```python
from build123d import *

# Parameters (mm, degrees)
CYLINDER017_R           = 1.4
CYLINDER017_DEPTH       = 210
CYLINDER017_PITCH_ANGLE = 90
CYLINDER016_R           = 1.4
CYLINDER016_DEPTH       = 16
CYLINDER016_PITCH_ANGLE = 90
CYLINDER022_R           = 1.4
CYLINDER022_DEPTH       = 210
CYLINDER022_PITCH_ANGLE = 90
CYLINDER011_R           = 1.4
CYLINDER011_DEPTH       = 140
CYLINDER018_R           = 1.4
CYLINDER018_DEPTH       = 16
CYLINDER013_R           = 1.4
CYLINDER013_DEPTH       = 140
CYLINDER020_R           = 1.4
CYLINDER020_DEPTH       = 16
CYLINDER014_R           = 1.4
CYLINDER014_DEPTH       = 140
CYLINDER019_R           = 1.4
CYLINDER019_DEPTH       = 16
CYLINDER021_R           = 1.4
CYLINDER021_DEPTH       = 16
CYLINDER012_R           = 1.4
CYLINDER012_DEPTH       = 140
CYLINDER015_R           = 1.4
CYLINDER015_DEPTH       = 210
CYLINDER015_PITCH_ANGLE = 90
CYLINDER002_R           = 12
CYLINDER002_DEPTH       = 40
BOX014_W                = 204
BOX014_H                = 20
BOX014_DEPTH            = 134
THICKNESS_T             = -6
FILLET007_R             = 3
BOX011_W                = 186
BOX011_H                = 34
BOX011_DEPTH            = 94
BOX010_W                = 192
BOX010_H                = 9
BOX010_DEPTH            = 122
BOX009_W                = 174
BOX009_H                = 10
BOX009_DEPTH            = 77
BOX012_W                = 192
BOX012_H                = 19
BOX012_DEPTH            = 21
BOX002_W                = 200
BOX002_H                = 40
BOX002_DEPTH            = 130
FILLET005_R             = 5
CYLINDER001_R           = 15
CYLINDER001_DEPTH       = 28
FILLET008_R             = 1
CHAMFER_SIZE            = 4
FILLET009_R             = 2


with BuildPart() as cylinder017:
    # Cylinder017 → Cylinder017 (new body)
    with BuildSketch(Plane.XY):
        Circle(CYLINDER017_R)
    extrude(amount=CYLINDER017_DEPTH)


with BuildPart() as cylinder017_1:
    # Cylinder017 pitch: moved
    add(cylinder017.part.rotate(Axis((0, 0, 0), (0, 1, 0)), CYLINDER017_PITCH_ANGLE))


with BuildPart() as cylinder017_2:
    # Cylinder017 placement: moved
    add(cylinder017_1.part.moved(Location((-5, 55, 65))))


with BuildPart() as cylinder016:
    # Cylinder016 → Cylinder016 (new body)
    with BuildSketch(Plane.XY):
        Circle(CYLINDER016_R)
    extrude(amount=CYLINDER016_DEPTH)


with BuildPart() as cylinder016_1:
    # Cylinder016 pitch: moved
    add(cylinder016.part.rotate(Axis((0, 0, 0), (0, 1, 0)), CYLINDER016_PITCH_ANGLE))


with BuildPart() as cylinder016_2:
    # Cylinder016 placement: moved
    add(cylinder016_1.part.moved(Location((-5, 55, 115))))


with BuildPart() as cylinder022:
    # Cylinder022 → Cylinder022 (new body)
    with BuildSketch(Plane.XY):
        Circle(CYLINDER022_R)
    extrude(amount=CYLINDER022_DEPTH)


with BuildPart() as cylinder022_1:
    # Cylinder022 pitch: moved
    add(cylinder022.part.rotate(Axis((0, 0, 0), (0, 1, 0)), CYLINDER022_PITCH_ANGLE))


with BuildPart() as cylinder022_2:
    # Cylinder022 placement: moved
    add(cylinder022_1.part.moved(Location((189, 55, 115))))


with BuildPart() as cylinder011:
    # Cylinder011 → Cylinder011 (new body)
    with BuildSketch(Plane(origin=(15, 55, 116), x_dir=(1, 0, 0), z_dir=(0, 0, 1))):
        Circle(CYLINDER011_R)
    extrude(amount=CYLINDER011_DEPTH)


with BuildPart() as cylinder018:
    # Cylinder018 → Cylinder018 (new body)
    with BuildSketch(Plane(origin=(15, 55, -5), x_dir=(1, 0, 0), z_dir=(0, 0, 1))):
        Circle(CYLINDER018_R)
    extrude(amount=CYLINDER018_DEPTH)


with BuildPart() as cylinder013:
    # Cylinder013 → Cylinder013 (new body)
    with BuildSketch(Plane(origin=(70, 55, 116), x_dir=(1, 0, 0), z_dir=(0, 0, 1))):
        Circle(CYLINDER013_R)
    extrude(amount=CYLINDER013_DEPTH)


with BuildPart() as cylinder020:
    # Cylinder020 → Cylinder020 (new body)
    with BuildSketch(Plane(origin=(125, 55, -5), x_dir=(1, 0, 0), z_dir=(0, 0, 1))):
        Circle(CYLINDER020_R)
    extrude(amount=CYLINDER020_DEPTH)


with BuildPart() as cylinder014:
    # Cylinder014 → Cylinder014 (new body)
    with BuildSketch(Plane(origin=(125, 55, 116), x_dir=(1, 0, 0), z_dir=(0, 0, 1))):
        Circle(CYLINDER014_R)
    extrude(amount=CYLINDER014_DEPTH)


with BuildPart() as cylinder019:
    # Cylinder019 → Cylinder019 (new body)
    with BuildSketch(Plane(origin=(70, 55, -5), x_dir=(1, 0, 0), z_dir=(0, 0, 1))):
        Circle(CYLINDER019_R)
    extrude(amount=CYLINDER019_DEPTH)


with BuildPart() as cylinder021:
    # Cylinder021 → Cylinder021 (new body)
    with BuildSketch(Plane(origin=(180, 55, -5), x_dir=(1, 0, 0), z_dir=(0, 0, 1))):
        Circle(CYLINDER021_R)
    extrude(amount=CYLINDER021_DEPTH)


with BuildPart() as cylinder012:
    # Cylinder012 → Cylinder012 (new body)
    with BuildSketch(Plane(origin=(180, 55, 116), x_dir=(1, 0, 0), z_dir=(0, 0, 1))):
        Circle(CYLINDER012_R)
    extrude(amount=CYLINDER012_DEPTH)


with BuildPart() as fusion009:
    # Cylinder015 → Cylinder015 (new body)
    with BuildSketch(Plane.XY):
        Circle(CYLINDER015_R)
    extrude(amount=CYLINDER015_DEPTH)


with BuildPart() as fusion009_1:
    # Cylinder015 pitch: moved
    add(fusion009.part.rotate(Axis((0, 0, 0), (0, 1, 0)), CYLINDER015_PITCH_ANGLE))


with BuildPart() as fusion009_2:
    # Cylinder015 placement: moved
    add(fusion009_1.part.moved(Location((-5, 55, 15))))

    # Fusion009: union Cylinder017, Cylinder016, Cylinder022, Cylinder011, Cylinder018, Cylinder013, Cylinder020, Cylinder014, Cylinder019, Cylinder021, Cylinder012
    add(cylinder017_2.part)
    add(cylinder016_2.part)
    add(cylinder022_2.part)
    add(cylinder011.part)
    add(cylinder018.part)
    add(cylinder013.part)
    add(cylinder020.part)
    add(cylinder014.part)
    add(cylinder019.part)
    add(cylinder021.part)
    add(cylinder012.part)


with BuildPart() as cylinder002:
    # Cylinder002 → Cylinder002 (new body)
    with BuildSketch(Plane(origin=(40, 70, 120), x_dir=(1, 0, 0), z_dir=(0, 0, 1))):
        Circle(CYLINDER002_R)
    extrude(amount=CYLINDER002_DEPTH)


with BuildPart() as fillet007:
    # Box014 → Box014 (new body)
    with BuildSketch(Plane(origin=(-2, 48, -2), x_dir=(1, 0, 0), z_dir=(0, 0, 1))):
        with Locations((102, 10)):
            Rectangle(BOX014_W, BOX014_H)
    extrude(amount=BOX014_DEPTH)

    # Thickness
    thickness_openings = [fillet007.faces().sort_by_distance(p)[0] for p in [
        (100, 48, 65),
        (100, 68, 65),
    ]]
    offset(amount=THICKNESS_T, openings=thickness_openings)

    # Fillet007
    fillet007_edges = [fillet007.edges().sort_by_distance(p)[0] for p in [
        (196, 58, 4),
        (4, 58, 4),
        (196, 58, 126),
        (4, 58, 126),
    ]]
    fillet(fillet007_edges, radius=FILLET007_R)


with BuildPart() as fillet007_1:
    # Fillet007 placement: moved
    add(fillet007.part.moved(Location((0, -8, 0))))


with BuildPart() as cube011:
    # Box011 → Box011 (new body)
    with BuildSketch(Plane(origin=(7, 45, 7), x_dir=(1, 0, 0), z_dir=(0, 0, 1))):
        with Locations((93, 17)):
            Rectangle(BOX011_W, BOX011_H)
    extrude(amount=BOX011_DEPTH)


with BuildPart() as cube010:
    # Box010 → Box010 (new body)
    with BuildSketch(Plane(origin=(4, 82, 4), x_dir=(1, 0, 0), z_dir=(0, 0, 1))):
        with Locations((96, 4.5)):
            Rectangle(BOX010_W, BOX010_H)
    extrude(amount=BOX010_DEPTH)


with BuildPart() as cube009:
    # Box009 → Box009 (new body)
    with BuildSketch(Plane(origin=(13, 75, 16), x_dir=(1, 0, 0), z_dir=(0, 0, 1))):
        with Locations((87, 5)):
            Rectangle(BOX009_W, BOX009_H)
    extrude(amount=BOX009_DEPTH)


with BuildPart() as fusion004:
    # Box012 → Box012 (new body)
    with BuildSketch(Plane(origin=(4, 67, 105), x_dir=(1, 0, 0), z_dir=(0, 0, 1))):
        with Locations((96, 9.5)):
            Rectangle(BOX012_W, BOX012_H)
    extrude(amount=BOX012_DEPTH)

    # Fusion004: union Cube011, Cube010, Cube009
    add(cube011.part)
    add(cube010.part)
    add(cube009.part)


with BuildPart() as fusion004_1:
    # Fusion004 placement: moved
    add(fusion004.part.moved(Location((0, -4, 0))))


with BuildPart() as cut009:
    # Box002 → Box002 (new body)
    with BuildSketch(Plane(origin=(0, 50, 0), x_dir=(1, 0, 0), z_dir=(0, 0, 1))):
        with Locations((100, 20)):
            Rectangle(BOX002_W, BOX002_H)
    extrude(amount=BOX002_DEPTH)

    # Fillet005
    fillet005_edges = [cut009.edges().sort_by_distance(p)[0] for p in [
        (0, 70, 130),
        (0, 90, 65),
        (0, 70, 0),
        (200, 70, 130),
        (200, 90, 65),
        (200, 70, 0),
        (100, 90, 0),
        (100, 90, 130),
    ]]
    fillet(fillet005_edges, radius=FILLET005_R)

    # Cut006: cut Fusion004
    add(fusion004_1.part, mode=Mode.SUBTRACT)

    # Cut009: cut Fillet007
    add(fillet007_1.part, mode=Mode.SUBTRACT)


with BuildPart() as fillet009:
    # Cylinder001 → Cylinder001 (new body)
    with BuildSketch(Plane(origin=(40, 70, 126), x_dir=(1, 0, 0), z_dir=(0, 0, 1))):
        Circle(CYLINDER001_R)
    extrude(amount=CYLINDER001_DEPTH)

    # Fusion008: union Cut009
    add(cut009.part)

    # Cut010: cut Cylinder002
    add(cylinder002.part, mode=Mode.SUBTRACT)

    # Cut012: cut Fusion009
    add(fusion009_2.part, mode=Mode.SUBTRACT)

    # Fillet008
    fillet008_edges = [fillet009.edges().sort_by_distance(p)[0] for p in [
        (25, 70, 154),
        (195.12132, 50, 125.12132),
    ]]
    fillet(fillet008_edges, radius=FILLET008_R)

    # Chamfer
    chamfer_edges = [fillet009.edges().sort_by_distance(p)[0] for p in [
        (40, 63, 120),
    ]]
    chamfer(chamfer_edges, length=CHAMFER_SIZE)

    # Fillet009
    fillet009_edges = [fillet009.edges().sort_by_distance(p)[0] for p in [
        (17.126603, 63, 126),
        (4, 63, 115.5),
        (100, 63, 105),
        (122.873397, 63, 126),
        (196, 63, 115.5),
        (4, 75, 126),
        (100, 87, 126),
        (196, 75, 126),
        (4, 78, 54.5),
        (4, 70.5, 105),
        (4, 87, 65),
        (4, 82.5, 4),
        (100, 78, 105),
        (196, 70.5, 105),
        (196, 78, 54.5),
        (196, 82.5, 4),
        (196, 87, 65),
        (100, 87, 4),
        (100, 78, 4),
    ]]
    fillet(fillet009_edges, radius=FILLET009_R)


solid = fillet009.part
```
Part model, mm, in its own coordinate system. A direction names the side the tool comes from. Round coordinates to 2 decimals unless told otherwise and drop trailing zeros. Order: outer loops, then holes, each group sorted by start corner. A loop starts at its lowest first (then second) coordinate and runs counter-clockwise, first axis right, second up. Notation, with made-up numbers: M 7.5,61 L 64.5,61 A6 cw 64.5,70 Z; hole C 86,-11 d2. An arc over 180 degrees is marked long. Answer in a Markdown table with one row per item. Add a question column.
Q1. Pin check, flat tips, straight feed: pin 1 (1.4 mm diameter, centred on y = 55.5, z = 115, fed in from +X); pin 2 (2 mm diameter, centred on y = 55, z = 15, fed in from +X); pin 3 (1 mm diameter, centred on y = 57.5, z = 23.5, fed in from -X); pin 4 (4.5 mm diameter, centred on x = 70, y = 55, fed in from -Z). Stop position of each tip, or through.
Q2. 3-axis set-ups, long thin cutter, end or side, ignore diameter. For faces 1 (the face through (99, 87, 64)), 2 (the face through (4, 56.4, 64.2)), 3 (the face through (37.399, 58.285, 138.956)): which of +Z, -Z, +X, -X, +Y, -Y reach the whole face in a straight line?
Q3. Mould opens along Y. For faces 4 (the face through (1, 88, 66)), 5 (the face through (93, 75, 15)), 6 (the face through (99, 71, 105)), 7 (the face through (1, 73, 128)) say: +Y half, -Y half, draft (parallel to the pull), parting line (faces both ways), or undercut.
Q4. Wall check: L1, parallel to Y at x = 180, z = 6.45; L2, parallel to X at y = 55, z = 123.25; L3, parallel to Y at x = 180, z = 123. Give the ranges that are in metal, low to high. Write a range as from..to.
Q5. Cut at A-A on z = 30. Give the cut face in (x, y), and give its area (3 significant figures).
Established:
| question | item | result |
|---|---|---|
| 1 | pin 1 | stops at x = 189 |
| 1 | pin 2 | passes through |
| 1 | pin 3 | stops at x = 4 |
| 1 | pin 4 | stops at z = 4 |
| 2 | face 1 | none |
| 2 | face 2 | +Z, -Z, -X, -Y |
| 2 | face 3 | +Z |
| 3 | face 4 | +Y half |
| 3 | face 5 | -Y half |
| 3 | face 6 | undercut |
| 3 | face 7 | draft |
| 4 | L1 | y = 50..53.6, 56.4..78, 87..90 |
| 4 | L2 | x = 4.01..13.6, 16.4..68.6, 71.4..123.6, 126.4..178.6, 181.4..195.99 |
| 4 | L3 | y = 50..53.6, 56.4..63, 87..90 |
| 5 | outline | M 0,60 L 4,60 L 4,51 A1 ccw 5,50 L 7,50 L 7,75 L 13,75 L 13,78 L 6,78 A2 cw 4,80 L 4,85 A2 cw 6,87 L 194,87 A2 cw 196,85 L 196,80 A2 cw 194,78 L 187,78 L 187,75 L 193,75 L 193,50 L 195,50 A1 ccw 196,51 L 196,60 L 200,60 L 200,85 A5 ccw 195,90 L 5,90 A5 ccw 0,85 Z |
| 5 | area | 1,010 mm2 |
